The model under review builds one solid part; all positions refer to its coordinate system, in mm. Face numbers are marked on the shaded views. Round coordinates to 2 decimals unless told otherwise and drop trailing zeros. Loops run counter-clockwise (first coordinate to the right, second up) from the corner with the lowest first, then second, coordinate; pieces in that order, holes last. Notation, with made-up numbers: M -11,59.5 L 48,59.5 A23 ccw 48,78.5 Z; hole C 26.25,41 d5. An arc over 180 degrees is marked long. Answer in a Markdown table with one row per item. Add a question column.
from build123d import *

# Parameters (mm, degrees)
F1_DEPTH = 25.4
F2_R     = 33.5189811659
F5_W     = 34.29
F5_H     = 2.286
F6_DEPTH = 22.225
F8_DEPTH = 0.1524


with BuildPart() as f1:
    # F0 (on Top) → F1 (new body)
    with BuildSketch(Plane.XY):
        with BuildLine():
            Line((0, -19.05), (0, 19.05))
            Line((0, 19.05), (-19.05, 19.05))
            ThreePointArc((-19.05, 19.05), (-38.1, 0), (-19.05, -19.05))
            Line((-19.05, -19.05), (0, -19.05))
        make_face()
    extrude(amount=F1_DEPTH)

    # F3: sweep along a path in F3_path
    with BuildLine(Plane(origin=(-19.05, -19.05, 25.4), x_dir=(0, 1, 0), z_dir=(0, 0, 1))) as f3_path:
        Line((0, -19.05), (0, 0))
        ThreePointArc((0, 0), (19.05, 19.05), (38.1, 0))
        Line((38.1, 0), (38.1, -19.05))
    # F2 (on Right) → F3 (sweep, cut)
    with BuildSketch(Plane.YZ):
        with Locations((-35.9534211457, 31.4643979073)):
            Circle(F2_R)
    sweep(path=f3_path.line, mode=Mode.SUBTRACT)

    # F4: F1 across face


with BuildPart() as f1_1:
    add(f1.part)
    add(f1.part.mirror(Plane(origin=(0, 0, 8.7269001071), x_dir=(0, 1, 0), z_dir=(1, 0, 0))))

    # F5 (on face) → F6 (cut)
    with BuildSketch(Plane.XY.offset(25.4)):
        Rectangle(F5_W, F5_H)
    extrude(amount=-F6_DEPTH, mode=Mode.SUBTRACT)

    # F7 (on face) → F8 (cut)
    with BuildSketch(Plane(origin=(0, 0, 0), x_dir=(1, 0, 0), z_dir=(0, 0, -1))):
        with BuildLine():
            ThreePointArc((19.05, -15.875), (34.925, 0), (19.05, 15.875))
            Line((19.05, 15.875), (-19.05, 15.875))
            ThreePointArc((-19.05, 15.875), (-34.925, 0), (-19.05, -15.875))
            Line((-19.05, -15.875), (19.05, -15.875))
        make_face()
    extrude(amount=-F8_DEPTH, mode=Mode.SUBTRACT)


solid = f1_1.part
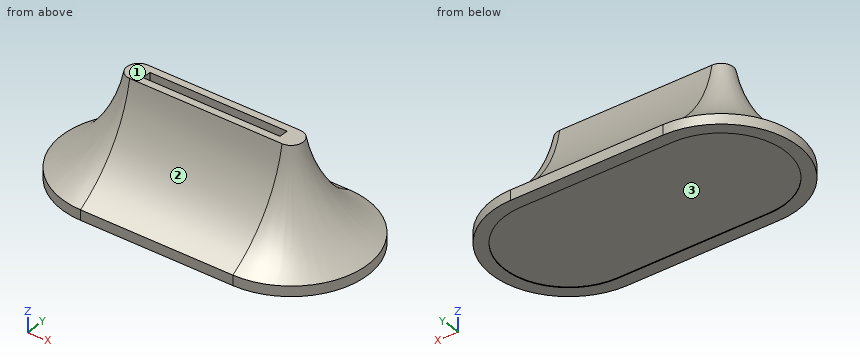
1. Take a section at D-D, the plane z = 13. State the section outline as (x, y) points (3 decimals), and give its area (3 significant figures).
2. Take a section at C-C, the plane x = -14.5. State the section outline as (y, z) points (3 decimals), and give its area (3 significant figures).
3. Take a section at A-A, the plane y = 0. State the section outline as (x, z) points (3 decimals), and give its area (3 significant figures).
4. To check wall thickness, follow probe 1 along Y at (x, z) = (-6, 20.75); probe 2 along Y at (x, z) = (11.5, 20.25); probe 3 along Z at (x, y) = (17.5, -1.5). State the ranges of each line that lie inside material, in increasing order.
5. Take a section at B-B, the plane z = 20. State the section outline as (x, y) points (3 decimals).
6. For pin 1 Ø9.5 at (x, y) = (9.5, 3.5) entering from -Z; pin 2 Ø6 at (x, z) = (10, 10) entering from -Y; pin 3 Ø3 at (x, z) = (-3.5, 21.5) entering from +Y; pin 4 Ø3 at (y, z) = (13.5, 10) entering from -X, all flat-tipped, find the tip position at first contact; note any pin that passes through.
7. Mouldability with a two-part tool opening along Y and no side actions: class the marked faces 1, 2 and 3 as released by +Y, released by -Y, zero draft, split by the parting line, or undercut.
Check sheet entries:
| question | item | result |
|---|---|---|
| 1 | outline | M -19.05,-7.979 L 19.05,-7.979 A7.979 ccw 19.05,7.979 L -19.05,7.979 A7.979 ccw Z; hole M -17.145,-1.143 L 17.145,-1.143 L 17.145,1.143 L -17.145,1.143 Z |
| 1 | area | 730 mm^2 |
| 2 | outline | M -19.05,0 L -15.875,0 L -15.875,0.152 L 15.875,0.152 L 15.875,0 L 19.05,0 L 19.05,2.52 A33.519 cw 2.988,25.4 L 1.143,25.4 L 1.143,3.175 L -1.143,3.175 L -1.143,25.4 L -2.988,25.4 A33.519 cw -19.05,2.52 Z |
| 2 | area | 430 mm^2 |
| 3 | outline | M -38.1,0 L -34.925,0 L -34.925,0.152 L 34.925,0.152 L 34.925,0 L 38.1,0 L 38.1,2.52 A33.519 cw 22.038,25.4 L 17.145,25.4 L 17.145,3.175 L -17.145,3.175 L -17.145,25.4 L -22.038,25.4 A33.519 cw -38.1,2.52 Z |
| 3 | area | 680 mm^2 |
| 4 | probe 1 | y = -4.19 to -1.14, 1.14 to 4.19 |
| 4 | probe 2 | y = -4.37 to -1.14, 1.14 to 4.37 |
| 4 | probe 3 | z = 0.15 to 25.4 |
| 5 | outline | M -19.05,-4.456 L 19.05,-4.456 A4.456 ccw 19.05,4.456 L -19.05,4.456 A4.456 ccw Z; hole M -17.145,-1.143 L 17.145,-1.143 L 17.145,1.143 L -17.145,1.143 Z |
| 6 | pin 1 | stops at z = 0.15 |
| 6 | pin 2 | stops at y = -13.04 |
| 6 | pin 3 | stops at y = 4.46 |
| 6 | pin 4 | passes through |
| 7 | face 1 | zero draft |
| 7 | face 2 | released by -Y |
| 7 | face 3 | undercut |
